Can you work these out from the drawing? Everything is in mm from the part's minimum corner. A direction names the side the tool comes from. Coordinates: 2 decimals unless noted, no trailing zeros. Write each loop counter-clockwise with the first axis right and the second up, starting at its lowest first coordinate (ties: lowest second). Pieces come first, ordered by that corner, then holes. Notation, with made-up numbers: M -7,12.5 L 42,12.5 A28 cw 42,39.5 Z; hole C 74,70 d6. An arc over 180 degrees is marked long. Write item = value, one per line.
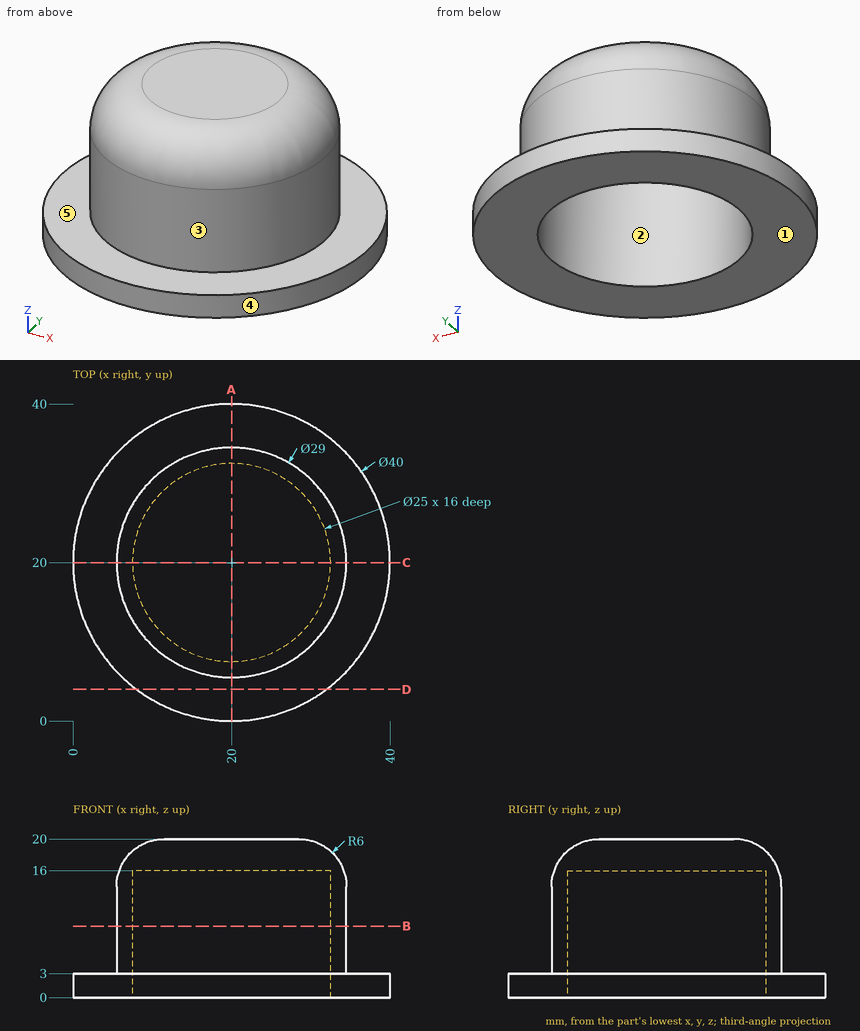
Item 1: Imagine slicing it at A-A (x = 20). Write out the boundary of the cut face in (y, z), and give its area (3 significant figures).
Numbers:
outline = M 0,0 L 7.5,0 L 7.5,16 L 32.5,16 L 32.5,0 L 40,0 L 40,3 L 34.5,3 L 34.5,14 A6 ccw 28.5,20 L 11.5,20 A6 ccw 5.5,14 L 5.5,3 L 0,3 Z
area = 198 mm²
Item 2: If I drill on line 1 along Y through (x, z) = (20, 5.5); line 2 along Z through (x, y) = (3, 29); line 3 along X through (y, z) = (31.5, 11), over which ranges is the centre line in solid material (lowest first)?
Numbers:
line_1 = 5.5 to 7.5, 32.5 to 34.5
line_2 = 0 to 3
line_3 = 11.17 to 15.1, 24.9 to 28.83
Item 3: If we mould it in two halves opening along Y, with no side actions, what happens to the marked faces 1, 2 and 3? For each: pulls with the +Y half, pulls with the -Y half, needs draft (parallel to the pull), parting line crosses it, or undercut.
Numbers:
face_1 = needs draft
face_2 = undercut
face_3 = parting line crosses it
Item 4: Imagine slicing it at D-D (y = 4). Write out the boundary of the cut face in (x, z).
Numbers:
outline = M 8,0 L 32,0 L 32,3 L 8,3 Z
Item 5: For the marked faces 4 and 5, which set-ups out of +Z, -Z, +X, -X, +Y, -Y let a thin tool reach every point of the face, with its end or its side?
Numbers:
face_4 = +Z, -Z
face_5 = +Z
Item 6: I'm going to push flat-ended pins straight in: P1, Ø6, axis at x = 10, z = 7.5, coming from the +Y side; P2, Ø12.5, axis at x = 17.5, y = 16, coming from the -Z side; P3, Ø12, axis at x = 17, z = 17, coming from the -Y side. Where does each tip first touch, or does it pass through?
Numbers:
P1 = 32.7
P2 = 16
P3 = 5.5
Item 7: Imagine slicing it at B-B (z = 9). Write out the boundary of the cut face in (x, y).
Numbers:
outline = C 20,20 d29; hole C 20,20 d25
